```python
from build123d import *

# Parameters (mm, degrees)
BOX058_W     = 4
BOX058_H     = 24
BOX058_DEPTH = 9.6
BOX057_W     = 4
BOX057_H     = 28.4
BOX057_DEPTH = 14


with BuildPart() as cube050:
    # Box058 → Box058 (new body)
    with BuildSketch(Plane(origin=(0, 2.2, 2.2), x_dir=(1, 0, 0), z_dir=(0, 0, 1))):
        with Locations((2, 12)):
            Rectangle(BOX058_W, BOX058_H)
    extrude(amount=BOX058_DEPTH)


with BuildPart() as obj1:
    # Box057 → Box057 (new body)
    with BuildSketch(Plane.XY):
        with Locations((2, 14.2)):
            Rectangle(BOX057_W, BOX057_H)
    extrude(amount=BOX057_DEPTH)

    # Cut053: cut Cube050
    add(cube050.part, mode=Mode.SUBTRACT)


with BuildPart() as obj1_1:
    # Cut053 placement: moved
    add(obj1.part.moved(Location((-4, 40.8, 32))))


solid = obj1_1.part
```
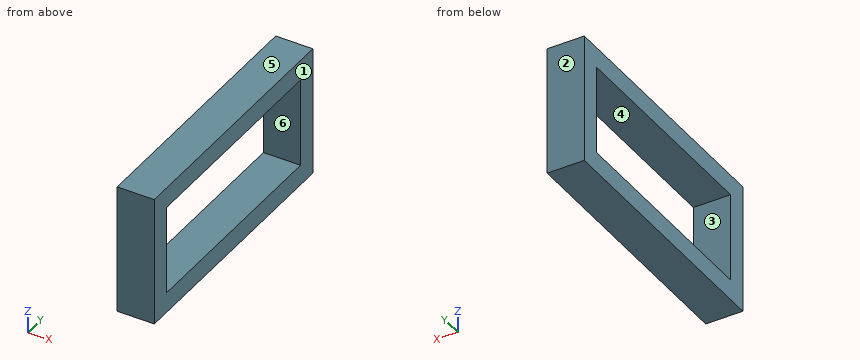
The model under review builds one solid part; all positions refer to its coordinate system, in mm. Face numbers are marked on the shaded views. A direction names the side the tool comes from. Give positions to 0.01 mm unless a question says otherwise; leave off trailing zeros. Write each loop counter-clockwise with the first axis right and the second up, starting at its lowest first coordinate (ties: lowest second). Pieces come first, ordered by that corner, then holes. Notation, with made-up numbers: (-15, -32.75) -> (-8, -32.75) arc R24 ccw to (-8, -15.75) -> close; hole circle Ø1 at (71.5, 60). An arc over 180 degrees is marked (long way). Answer in a Markdown table with one row per item.
1) Add section C-C on x = -0.35. State the section outline as (y, z) points.
Worked answers:
| item | result |
|---|---|
| outline | (40.8, 32) -> (69.2, 32) -> (69.2, 46) -> (40.8, 46) -> close; hole (43, 34.2) -> (67, 34.2) -> (67, 43.8) -> (43, 43.8) -> close |
2) Tool access review of the marked faces 5 and 6: name each direction out of +Z, -Z, +X, -X, +Y, -Y from which nothing blocks a thin tool from reaching the whole face with its end or side.
Worked answers:
| item | result |
|---|---|
| face 5 | +Z, +X, -X, +Y, -Y |
| face 6 | +X, -X |
3) For L1, parallel to Z at x = -2.6, y = 58; L2, parallel to Y at x = -3.4, z = 37.5, list the stretches that pass through material, from the lowest coordinate up. Write a range as [from, to].
Worked answers:
| item | result |
|---|---|
| L1 | [32, 34.2], [43.8, 46] |
| L2 | [40.8, 43], [67, 69.2] |
4) Add section A-A on z = 42.5. State the section outline as (x, y) points.
Worked answers:
| item | result |
|---|---|
| outline | (-4, 40.8) -> (0, 40.8) -> (0, 43) -> (-4, 43) -> close; (-4, 67) -> (0, 67) -> (0, 69.2) -> (-4, 69.2) -> close |
5) Mouldability with a two-part tool opening along Y and no side actions: class the marked faces 1, 2, 3 and 4 as +Y half, -Y half, draft (parallel to the pull), parting line (faces both ways), or undercut.
Worked answers:
| item | result |
|---|---|
| face 1 | draft |
| face 2 | +Y half |
| face 3 | undercut |
| face 4 | undercut |
6) Clearance check with a flat-ended pin moving along its axis: P1, Ø2, axis at y = 45, z = 38, coming from the +X side. State where the tip first meets the part, or that it passes through.
Worked answers:
| item | result |
|---|---|
| P1 | through |
7) Add section B-B on y = 58.75. State the section outline as (x, z) points.
Worked answers:
| item | result |
|---|---|
| outline | (-4, 32) -> (0, 32) -> (0, 34.2) -> (-4, 34.2) -> close; (-4, 43.8) -> (0, 43.8) -> (0, 46) -> (-4, 46) -> close |
